Source: CAD feature listing. Evaluate the final solid. Frame: model axes, mm. A direction names the side the tool comes from. Coordinates: 2 decimals unless noted, no trailing zeros. Write each loop counter-clockwise with the first axis right and the second up, starting at its lowest first coordinate (ties: lowest second). Pieces come first, ordered by that corner, then holes. Notation, with made-up numbers: M -19.5,71.25 L -2.5,71.25 A28 ccw -2.5,106.25 Z; hole C 50.25,-12.5 d9. An arc over 180 degrees is marked long. One line per item, written item: value. Start each with the question number.
Item 1: Cut plane D-D, the plane y = 40. Output: boundary loops of the cut face in (x, z), then the cut area to 3 significant figures.
Item 2: Cut plane C-C, the plane x = 28.5. Output: boundary loops of the cut face in (y, z).
Item 3: Set-up query: faces 1 (the flat face through (-5, 40, 5.08)), 2 (the flat face through (-31.75, 46, 3)), 3 (the flat face through (-12.7, 41, 3)). Return all of +Z, -Z, +X, -X, +Y, -Y with unobstructed straight access to the full face (end or side cutting, diameter ignored); none if empty.
Item 4: Cut plane B-B, the plane y = 0. Output: boundary loops of the cut face in (x, z) (3 decimals).
Item 5: Ray query, L1, parallel to X at y = 44.5, z = 2.05; L2, parallel to X at y = 0, z = 2.35 (3 decimals); L3, parallel to X at y = 35.5, z = 4.6. Return the intervals inside material, ascending. Write a range as from..to.
Item 6: Cut plane A-A, the plane z = 1.9. Output: boundary loops of the cut face in (x, y) (3 decimals).
Item 7: Pin query (flat end, axial travel): P1, Ø1.5, axis at x = -13, y = 33.5, coming from the -Z side; P2, Ø1, axis at x = 0.5, z = 4, coming from the -Y side; P3, Ø2.5, axis at y = 45.5, z = 2, coming from the +X side; P4, Ø1.5, axis at y = 42, z = 3, coming from the -X side. Return the tip coordinate at first contact, or that it passes through.
Item 8: Mould query, pull axis Y, two halves, no side actions, for faces 4 (the flat face through (-10, 63.5, 3)), 5 (the flat face through (-10, 31.75, 3)), 6 (the cylindrical face through (32.14, 13.67, 2.5)), 7 (the flat face through (30, -12.7, 3)). Classes: released by +Y, released by -Y, zero draft, split by the parting line, or undercut.
```python
from build123d import *

# Parameters (mm, degrees)
SKETCH1_R           = 34.925
BOSS_EXTRUDE1_DEPTH = 5.08
SKETCH2_W           = 25.4
SKETCH2_H           = 5.08
BOSS_EXTRUDE2_DEPTH = 63.5
SKETCH3_R           = 29.972
CUT_EXTRUDE1_DEPTH  = 50.8
SKETCH4_W           = 5.08
SKETCH4_H           = 19.05
CUT_EXTRUDE2_DEPTH  = 50.8
SKETCH5_W           = 129.040366972
SKETCH5_H           = 73.118289239
CUT_EXTRUDE3_DEPTH  = 50.8
SKETCH6_W           = 5.08
SKETCH6_H           = 34.29
BOSS_EXTRUDE3_DEPTH = 19.05
SKETCH7_W           = 5.08
SKETCH7_H           = 19.05
CUT_EXTRUDE4_DEPTH  = 19.05
FILLET1_R           = 12.7


with BuildPart() as part:
    # Sketch1 → Boss-Extrude1 (new body)
    with BuildSketch(Plane.XY):
        Circle(SKETCH1_R)
    extrude(amount=BOSS_EXTRUDE1_DEPTH)

    # Sketch2 → Boss-Extrude2 (add)
    with BuildSketch(Plane(origin=(0, 0, 0), x_dir=(1, 0, 0), z_dir=(0, 1, 0))):
        with Locations((0, -2.54)):
            Rectangle(SKETCH2_W, SKETCH2_H)
    extrude(amount=BOSS_EXTRUDE2_DEPTH)

    # Sketch3 → Cut-Extrude1 (cut)
    with BuildSketch(Plane(origin=(0, 0, 0), x_dir=(-1, 0, 0), z_dir=(0, 0, -1))):
        Circle(SKETCH3_R)
    extrude(amount=-CUT_EXTRUDE1_DEPTH, mode=Mode.SUBTRACT)

    # Sketch4 → Cut-Extrude2 (cut)
    with BuildSketch(Plane(origin=(0, 0, 0), x_dir=(-1, 0, 0), z_dir=(0, 0, -1))):
        with Locations((0, 41.275)):
            Rectangle(SKETCH4_W, SKETCH4_H)
    extrude(amount=-CUT_EXTRUDE2_DEPTH, mode=Mode.SUBTRACT)

    # Sketch5 → Cut-Extrude3 (cut)
    with BuildSketch(Plane(origin=(0, 0, 0), x_dir=(-1, 0, 0), z_dir=(0, 0, -1))):
        with Locations((0.982448892, -49.25914462)):
            Rectangle(SKETCH5_W, SKETCH5_H)
    extrude(amount=-CUT_EXTRUDE3_DEPTH, mode=Mode.SUBTRACT)

    # Sketch6 → Boss-Extrude3 (add)
    with BuildSketch(Plane.ZY.offset(12.7)):
        with Locations((2.54, 46.355)):
            Rectangle(SKETCH6_W, SKETCH6_H)
    extrude(amount=BOSS_EXTRUDE3_DEPTH)

    # Sketch7 → Cut-Extrude4 (cut)
    with BuildSketch(Plane(origin=(0, 0, 0), x_dir=(-1, 0, 0), z_dir=(0, 0, -1))):
        with Locations((10.16, 41.275)):
            Rectangle(SKETCH7_W, SKETCH7_H)
    extrude(amount=-CUT_EXTRUDE4_DEPTH, mode=Mode.SUBTRACT)

    # Fillet1
    # the kernel refuses this fillet: 12.7 mm, written as the material it takes off along each edge
    with BuildSketch(Plane(origin=(12.7, 63.5, -31.75), x_dir=(-1, 0, 0), z_dir=(0, 0, 1))) as fillet1_piece_1:
        with BuildLine():
            CenterArc((FILLET1_R, FILLET1_R), FILLET1_R, 180, 90)
            Line((0, FILLET1_R), (0, 0))
            Line((0, 0), (FILLET1_R, 0))
        make_face()
    extrude(amount=68.58, mode=Mode.SUBTRACT)
    with BuildSketch(Plane(origin=(-31.75, 63.5, -31.75), x_dir=(1, 0, 0), z_dir=(0, 0, 1))) as fillet1_piece_2:
        with BuildLine():
            CenterArc((FILLET1_R, -FILLET1_R), FILLET1_R, 90, 90)
            Line((0, -FILLET1_R), (0, 0))
            Line((0, 0), (FILLET1_R, 0))
        make_face()
    extrude(amount=68.58, mode=Mode.SUBTRACT)
    with BuildSketch(Plane(origin=(-31.75, 29.21, 36.83), x_dir=(0, 1, 0), z_dir=(0, 0, -1))) as fillet1_piece_3_section:
        with BuildLine():
            CenterArc((FILLET1_R, FILLET1_R), FILLET1_R, 180, 90)
            Line((0, FILLET1_R), (0, 0))
            Line((0, 0), (FILLET1_R, 0))
        make_face()
    fillet1_piece_3 = extrude(amount=68.58, mode=Mode.PRIVATE)
    fillet1_piece_3 = fillet1_piece_3 - Plane(origin=(0, 0, 2.54), x_dir=(1, 0, 0), z_dir=(0, 0, -1)) * Cylinder(34.925, 188, mode=Mode.PRIVATE)
    add(fillet1_piece_3, mode=Mode.SUBTRACT)


solid = part.part
```
From the geometry:
1. outline: M -31.61,0 L -12.7,0 L -12.7,5.08 L -31.61,5.08 Z; M -7.62,0 L -2.54,0 L -2.54,5.08 L -7.62,5.08 Z; M 2.54,0 L 12.7,0 L 12.7,5.08 L 2.54,5.08 Z
1. area: 173 mm²
2. outline: M -12.7,0 L -9.28,0 L -9.28,5.08 L -12.7,5.08 Z; M 9.28,0 L 20.19,0 L 20.19,5.08 L 9.28,5.08 Z
3. face 1: +Z, +X, -X, +Y, -Y
3. face 2: +Z, -Z, -X, +Y
3. face 3: +Z, -Z
4. outline: M -34.925,0 L -29.972,0 L -29.972,5.08 L -34.925,5.08 Z; M 29.972,0 L 34.925,0 L 34.925,5.08 L 29.972,5.08 Z
5. L1: x = -31.75..-12.7, -7.62..-2.54, 2.54..12.7
5. L2: x = -34.925..-29.972, 29.972..34.925
5. L3: x = -30.01..-12.7, -7.62..-2.54, 2.54..12.7
6. outline: M -32.534,-12.7 L -27.148,-12.7 A29.972 cw long 27.148,-12.7 L 32.534,-12.7 A34.925 ccw 12.7,32.534 L 12.7,50.8 A12.7 ccw 0,63.5 L -19.05,63.5 A12.7 ccw -31.75,50.8 L -31.75,41.91 A12.7 ccw -19.144,29.21 A34.925 ccw Z; hole M -12.7,31.75 L -7.62,31.75 L -7.62,50.8 L -12.7,50.8 Z; hole M -2.54,31.75 L 2.54,31.75 L 2.54,50.8 L -2.54,50.8 Z
7. P1: stops at z = 0
7. P2: stops at y = 29.96
7. P3: stops at x = 12.7
7. P4: stops at x = -31.75
8. face 4: released by +Y
8. face 5: undercut
8. face 6: split by the parting line
8. face 7: released by -Y
